Input: part model. Units: mm. Frame: model coordinates. A direction names the side the tool comes from. Coordinates: 2 decimals unless noted, no trailing zeros. Loops run counter-clockwise (first coordinate to the right, second up) from the corner with the lowest first, then second, coordinate; pieces in that order, holes last. Notation, with made-up numbers: (-10.5, 57) - (47.5, 57) arc R25 ccw to (47.5, 80) - close; hole circle Ø11 at (5.5, -37). An arc over 180 degrees is marked (long way). Use a Markdown table: item, result. Add a question column.
1. Section query B-B on z = 1.6. Return the cut outline in (x, y), then the cut area to 3 significant figures.
2. Section query A-A on y = 18. Return the cut outline in (x, z), then the cut area to 3 significant figures.
3. Draft query along X for faces 1 (the face through (-14.96, 13.48, 0.97)), 2 (the face through (10, 5, 3)), 3 (the face through (42.499, 11.958, 0.972)), 4 (the face through (-14.172, 10.027, 0.972)). Return one class per face: released by +X, released by -X, zero draft, split by the parting line, or undercut.
4. Ray query, L1, parallel to Y at x = -10.5, z = -0.6; L2, parallel to X at y = -6, z = 0.7; L3, parallel to X at y = -3, z = -0.7. Return the intervals inside material, ascending. Write a range as [from, to].
5. Access query for faces 5 (the face through (-9, 15.434, 1)), 6 (the face through (-2.52, 3.45, 0.97)), 7 (the face through (-15.833, 2.595, 0.972)). Directions: +Z, -Z, +X, -X, +Y, -Y. A direction counts if a zero-diameter tool reaches every point of the face in a straight line with its end or side. Return the directions, or none.
6. Section query D-D on x = 28. Return the cut outline in (y, z).
7. Section query C-C on x = 2.5. Return the cut outline in (y, z).
8. Contact query for flat-ended pins moving along their axis: P1, Ø5.5, axis at x = 46.42, y = 16.21, coming from the +Z side; P2, Ø2, axis at x = 38, z = 2.5, coming from the -Y side; P3, Ø1.2, axis at x = -8.5, z = 0.5, coming from the +Y side. Output: stop coordinate, or through.
```python
from build123d import *

# Parameters (mm, degrees)
SKETCH2_R           = 1.75
BOSS_EXTRUDE1_DEPTH = 2
SCALE1_SCALE        = 2


with BuildPart() as part:
    # Sketch2 → Boss-Extrude1 (new body)
    with BuildSketch(Plane.XY):
        with BuildLine():
            Line((-2.959686812, 7.094235734), (-2.589510897, -0.112410482))
            ThreePointArc((-2.589510897, -0.112410482), (-1.732883601, -1.97439389), (0.17059178, -2.73437679))
            Line((0.17059178, -2.73437679), (9.218440829, -2.341769901))
            Line((9.218440829, -2.341769901), (22.318004544, 8.181471599))
            ThreePointArc((22.318004544, 8.181471599), (23.631672458, 8.589402593), (25.00585725, 8.528187863))
            Line((25.00585725, 8.528187863), (27.810968992, 7.908802431))
            ThreePointArc((27.810968992, 7.908802431), (30.836871293, 10.605873355), (27.325176398, 12.630293092))
            Line((27.325176398, 12.630293092), (13.285071523, 6.320301234))
            ThreePointArc((13.285071523, 6.320301234), (11.630616958, 5.968797328), (9.978797309, 6.332482295))
            Line((9.978797309, 6.332482295), (2.062383287, 9.960674362))
            Line((2.062383287, 9.960674362), (-0.662699736, 9.960674362))
            ThreePointArc((-0.662699736, 9.960674362), (-2.356294969, 8.964265917), (-2.959686812, 7.094235734))
        make_face()
        Circle(SKETCH2_R, mode=Mode.SUBTRACT)
        with Locations((28.35, 10.35)):
            Circle(SKETCH2_R, mode=Mode.SUBTRACT)
        with BuildLine():
            Line((-0.197115754, 5.55), (0, 5.55))
            ThreePointArc((0, 5.55), (3.924442636, 3.924442636), (5.55, 0))
            ThreePointArc((5.55, 0), (7.317827511, -1.749909192), (9.049636777, 0.035653171))
            ThreePointArc((9.049636777, 0.035653171), (6.258630387, 6.536569638), (-0.357350166, 9.042648827))
            ThreePointArc((-0.357350166, 9.042648827), (-1.945276995, 7.219798525), (-0.197115754, 5.55))
        make_face(mode=Mode.SUBTRACT)
    extrude(amount=BOSS_EXTRUDE1_DEPTH)


with BuildPart() as part_1:
    # Scale1: scaled about (10.278907769, 4.487421788, 1)
    add(part.part.scale(SCALE1_SCALE).moved(Location((-10.278907769, -4.487421788, -1))))


solid = part_1.part
```
Resolved:
| question | item | result |
|---|---|---|
| 1 | outline | (-16.2, 9.7) - (-15.46, -4.71) arc R5.53 ccw to (-9.94, -9.96) - (8.16, -9.17) - (34.36, 11.88) arc R8 cw to (39.73, 12.57) - (45.34, 11.33) arc R5 ccw (long way) to (44.37, 20.77) - (16.29, 8.15) arc R8 cw to (9.68, 8.18) - (-6.15, 15.43) - (-11.6, 15.43) arc R5.53 ccw to start; hole circle Ø7 at (-10.28, -4.49); hole (-10.99, 13.6) arc R3.5 ccw to (-10.67, 6.61) - (-10.28, 6.61) arc R11.1 cw to (0.82, -4.49) arc R3.5 ccw (long way) to (7.82, -4.42) arc R18.1 ccw to start; hole circle Ø7 at (46.42, 16.21) |
| 1 | area | 634 mm² |
| 2 | outline | (38.2, -1) - (43.41, -1) - (43.41, 3) - (38.2, 3) - close; (49.43, -1) - (51.09, -1) - (51.09, 3) - (49.43, 3) - close |
| 2 | area | 27.5 mm² |
| 3 | face 1 | released by -X |
| 3 | face 2 | zero draft |
| 3 | face 3 | undercut |
| 3 | face 4 | undercut |
| 4 | L1 | [-9.93, -7.98], [-0.99, 6.61], [13.61, 15.43] |
| 4 | L2 | [-15.24, -13.44], [-7.12, 1.16], [7.48, 12.11] |
| 4 | L3 | [-15.55, -13.45], [-7.11, 0.72], [7.76, 15.84] |
| 5 | face 5 | +Z, -Z, -X, +Y |
| 5 | face 6 | +Z, -Z |
| 5 | face 7 | +Z, -Z, -X, -Y |
| 6 | outline | (6.77, -1) - (13.42, -1) - (13.42, 3) - (6.77, 3) - close |
| 7 | outline | (-9.42, -1) - (-7.48, -1) - (-7.48, 3) - (-9.42, 3) - close; (8.33, -1) - (11.47, -1) - (11.47, 3) - (8.33, 3) - close |
| 8 | P1 | through |
| 8 | P2 | y = 12.69 |
| 8 | P3 | y = 15.43 |
